Print and shaded views of the part. All mm, measured from the part's lowest x, y and z. A direction names the side the tool comes from. Give positions to 0.01 mm unless a question says otherwise; leave off trailing zeros. Loops run counter-clockwise (first coordinate to the right, second up) from the corner with the lowest first, then second, coordinate; pieces in that order, holes last. Notation, with made-up numbers: (73.25, 7.25) -> (128.25, 7.25) arc R22 cw to (128.25, 42.25) -> close; hole circle Ø1 at (38, 82.5). An arc over 180 degrees is marked (long way). Write each question's results on one line, items separated by ' | '. Start each with the question number.
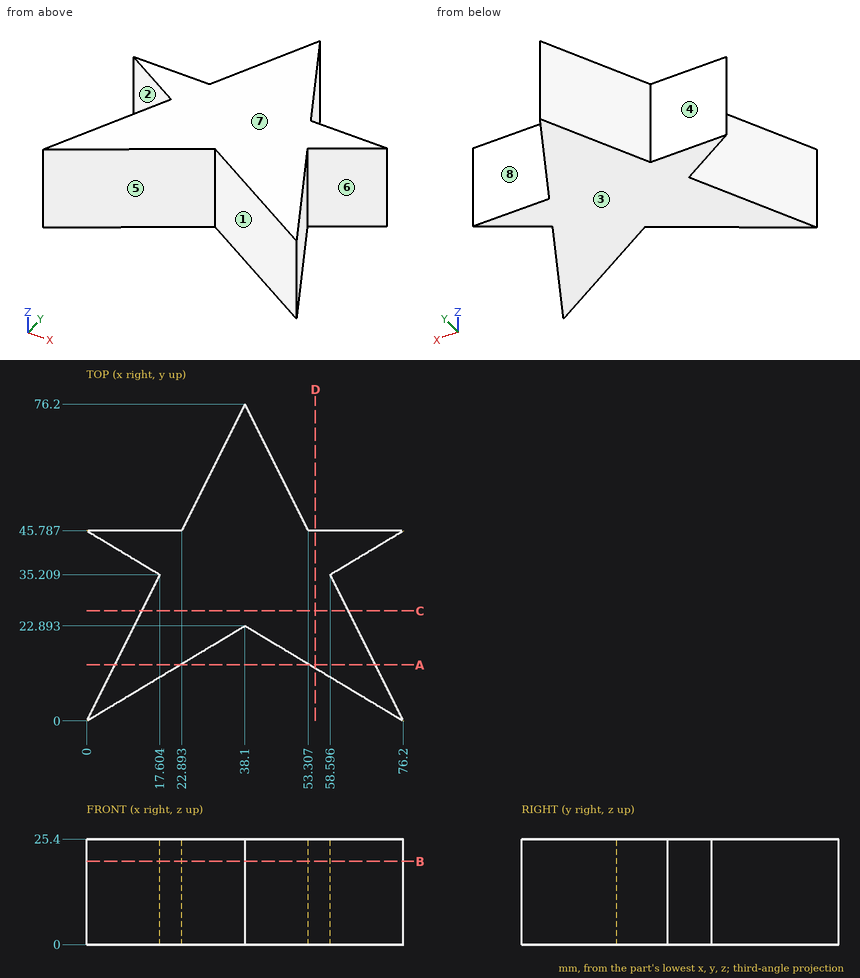
Q1. Saw through at D-D, the plane x = 55. List the corners of the cut face in (y, z).
Q2. Saw through at C-C, the plane y = 26.5. List the corners of the cut face in (x, z).
Q3. Saw through at A-A, the plane y = 13.5. List the corners of the cut face in (x, z).
Q4. Drop flat-ended pins along their axis: pin 1 (11.5 mm diameter, centred on x = 61, z = 17.5, fed in from +Y); pin 2 (8 mm diameter, centred on y = 35, z = 19, fed in from +X) (1 decimal); pin 3 (1 mm diameter, centred on x = 9.5, z = 3, fed in from -Y). Give the stop position or say it passes through.
Q5. Saw through at B-B, the plane z = 20. List the corners of the cut face in (x, y) (1 decimal), then the cut area to 3 significant figures.
Q6. Which spindle directions (+Z, -Z, +X, -X, +Y, -Y) get a long thin tool onto all of the face, cutting with end or side? Do the marked faces 1, 2, 3 and 4. Say none if no direction does.
Q7. Mould opens along Y. For the marked faces 5, 6, 7 and 8 say: pulls with the +Y half, pulls with the -Y half, needs draft (parallel to the pull), parting line crosses it, or undercut.
Q8. Wall check: L1, parallel to Y at x = 8, z = 23 (1 decimal); L2, parallel to Y at x = 15.5, z = 13 (1 decimal); L3, parallel to X at y = 65, z = 10.25. Give the ranges that are in metal, low to high.
Answer block:
1) outline: (12.74, 0) -> (45.79, 0) -> (45.79, 25.4) -> (12.74, 25.4) -> close
2) outline: (13.25, 0) -> (62.95, 0) -> (62.95, 25.4) -> (13.25, 25.4) -> close
3) outline: (6.75, 0) -> (22.47, 0) -> (22.47, 25.4) -> (6.75, 25.4) -> close; (53.73, 0) -> (69.45, 0) -> (69.45, 25.4) -> (53.73, 25.4) -> close
4) pin 1: stops at y = 45.79 | pin 2: stops at x = 64.9 | pin 3: stops at y = 5.41
5) outline: (0, 0) -> (38.1, 22.9) -> (76.2, 0) -> (58.6, 35.2) -> (76.2, 45.8) -> (53.3, 45.8) -> (38.1, 76.2) -> (22.9, 45.8) -> (0, 45.8) -> (17.6, 35.2) -> close | area: 2,270 mm2
6) face 1: +Z, -Z, -Y | face 2: +Z, -Z, -X | face 3: -Z, +X, -X, +Y, -Y | face 4: +Z, -Z, -X, +Y
7) face 5: pulls with the -Y half | face 6: undercut | face 7: needs draft | face 8: pulls with the +Y half
8) L1: y = 4.8 to 16, 41 to 45.8 | L2: y = 9.3 to 31, 36.5 to 45.8 | L3: x = 32.5 to 43.7
